Study the drawing (mm; zero at the part's minimum x, y, z) and answer. A direction names the side the tool comes from. Round coordinates to 2 decimals unless told otherwise and drop trailing zeros. Order: outer loops, then holes, each group sorted by start corner. A loop starts at its lowest first (then second) coordinate and runs counter-clockwise, first axis right, second up. Notation, with made-up numbers: (29, 16) - (45, 16) arc R17 ccw to (45, 33) - close; hole circle Ø2 at (21, -29.5). An arc over 180 degrees is marked (long way). Put each result on its own line as item: value. Start each with the question number.
Q1. Section B-B on x = 15 is taken. Give the vertices of the cut face in (y, z).
Q2. Find the intervals of material crossed by line 1 along Y through (x, z) = (6.75, 25.25); line 2 along Y through (x, z) = (13, 18.25); line 3 along Z through (x, y) = (15, 23), in increasing order. Write a range as from..to.
Q3. Each of these flat-tipped pins is pushed along its axis until it touches: pin 1 Ø5 at (y, z) = (15, 13.5) entering from +X; pin 2 Ø2 at (y, z) = (45, 15.5) entering from +X; pin 3 Ø10 at (y, z) = (29.5, 6) entering from +X; pin 4 Ø2 at (y, z) = (37, 23.5) entering from +X. Where does it stop, or does it pass through?
Q4. Section D-D on z = 22 is taken. Give the vertices of the cut face in (x, y).
Q5. Section C-C on x = 18.5 is taken. Give the vertices of the cut face in (y, z).
Q6. Which of the six approach directions +Z, -Z, +X, -X, +Y, -Y give full straight-line access (tool end or side, diameter ignored) to the marked faces 1, 2, 3, 4 and 5?
Q7. Section A-A on z = 15 is taken. Give the vertices of the cut face in (x, y).
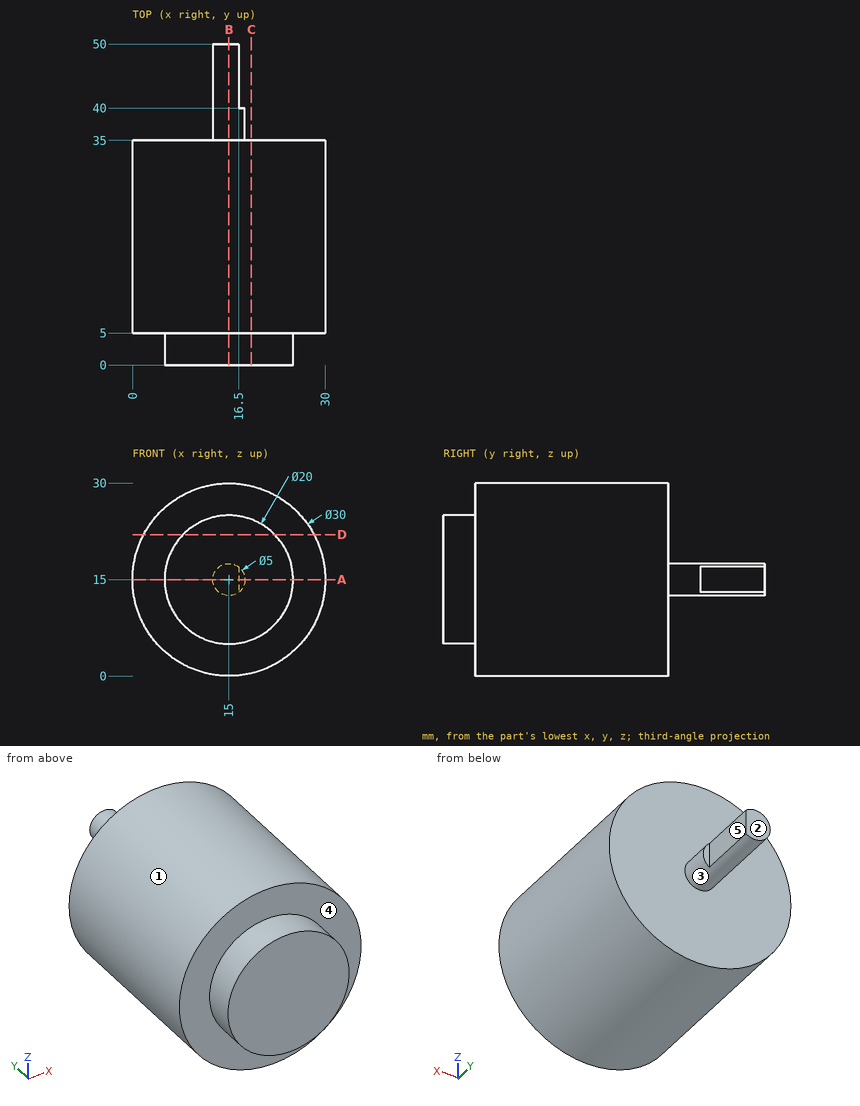
Findings:
1. outline: (0, 5) - (5, 5) - (5, 0) - (35, 0) - (35, 12.5) - (50, 12.5) - (50, 17.5) - (35, 17.5) - (35, 30) - (5, 30) - (5, 25) - (0, 25) - close
2. line 1: 5..35
2. line 2: 0..35
2. line 3: 0..30
3. pin 1: x = 30
3. pin 2: x = 16.5
3. pin 3: x = 29.46
3. pin 4: through
4. outline: (1.73, 5) - (7.86, 5) - (7.86, 0) - (22.14, 0) - (22.14, 5) - (28.27, 5) - (28.27, 35) - (1.73, 35) - close
5. outline: (0, 5.63) - (5, 5.63) - (5, 0.41) - (35, 0.41) - (35, 29.59) - (5, 29.59) - (5, 24.37) - (0, 24.37) - close
6. face 1: +Y, -Y
6. face 2: +Z, -Z, +X, -X, +Y
6. face 3: +Y
6. face 4: -Y
6. face 5: +Z, -Z, +X, +Y
7. outline: (0, 5) - (5, 5) - (5, 0) - (25, 0) - (25, 5) - (30, 5) - (30, 35) - (17.5, 35) - (17.5, 40) - (16.5, 40) - (16.5, 50) - (12.5, 50) - (12.5, 35) - (0, 35) - close
